For this review, take the finished solid that the model builds, in its own axes (mm). A direction names the side the tool comes from. Coordinates: 2 decimals unless noted, no trailing zeros. Order: outer loops, then holes, each group sorted by start corner. A loop starts at its lowest first (then second) coordinate and runs counter-clockwise, first axis right, second up. Notation, with made-up numbers: M 8.25,-24.75 L 24.25,-24.75 A18 ccw 24.25,-4.75 Z; hole C 19.25,-16 d10. An arc over 180 degrees is marked long. Use one line per item in the form item = value. Start each with the question number.
```python
from build123d import *

# Parameters (mm, degrees)
BOSS_EXTRUDE1_DEPTH = 15
BOSS_EXTRUDE2_DEPTH = 15
SKETCH3_W           = 12
SKETCH3_H           = 4.2
BOSS_EXTRUDE3_DEPTH = 15
CUT_EXTRUDE1_REACH  = 69
SKETCH4_R           = 3.15


with BuildPart() as part:
    # Sketch1 → Boss-Extrude1 (new body)
    with BuildSketch(Plane.XY):
        Polygon((-15, -15), (-15, -4.085), (-13, -2.085), (-17, -2.085), (-17, -17), (17, -17), (17, -2.085), (13, -2.085), (13, -4.085), (15, -4.085), (15, -15), align=None)
    extrude(amount=BOSS_EXTRUDE1_DEPTH)

    # Sketch2 → Boss-Extrude2 (add)
    with BuildSketch(Plane(origin=(0, 0, 0), x_dir=(-1, 0, 0), z_dir=(0, 0, -1))):
        Polygon((-80, 50), (-17, -2.085), (-17, -4.68000212), (-48.089133488, 21.022815621), (-51.622859883, 16.748556949), (-17, -14.313094489), (-17, -17), (-87, 45.8), (-87, 50), (-85, 50), (-85, 45.8), (-84, 45.8), (-84, 50), align=None)
        Polygon((-80.719691535, 48), (-49.630558047, 22.297182259), (-53.112776785, 18.085225255), (-82, 44.001191225), (-82, 48), align=None, mode=Mode.SUBTRACT)
    extrude(amount=-BOSS_EXTRUDE2_DEPTH)

    # Sketch3 → Boss-Extrude3 (add)
    with BuildSketch(Plane(origin=(0, 0, 0), x_dir=(-1, 0, 0), z_dir=(0, 0, -1))):
        with Locations((-93, 47.9)):
            Rectangle(SKETCH3_W, SKETCH3_H)
    extrude(amount=-BOSS_EXTRUDE3_DEPTH)

    # Sketch4 → Cut-Extrude1 (cut, up to next)
    with BuildSketch(Plane(origin=(0, 50, 0), x_dir=(1, 0, 0), z_dir=(0, 1, 0)), mode=Mode.PRIVATE) as cut_extrude1_sk1:
        with Locations((93, -7.5)):
            Circle(SKETCH4_R)
    cut_extrude1_tool1 = extrude(cut_extrude1_sk1.sketch, amount=-CUT_EXTRUDE1_REACH, mode=Mode.PRIVATE) & part.part
    add(cut_extrude1_tool1.solids().sort_by_distance((93, 50, 7.5))[0], mode=Mode.SUBTRACT)


solid = part.part
```
1. For pin 1 Ø3.5 at (y, z) = (-7.5, 4) entering from +X; pin 2 Ø2 at (x, z) = (15.5, 5) entering from +Y (3 decimals); pin 3 Ø8 at (y, z) = (13, 8) entering from -X, all flat-tipped, find the tip position at first contact; note any pin that passes through.
2. To check wall thickness, follow line 1 (Z direction, x = 93, y = 46.7); line 2 (X direction, y = 47.8, z = 7.5); line 3 (X direction, y = 49.1, z = 7.5). State the ranges of each line that lie inside material, in increasing order.
3. The part is to be moulded in two halves that separate along Z. For faces 1 (the flat face through (82, 50, 7)), 2 (the cylindrical face through (89.853, 47.929, 7.362)), 3 (the flat face through (41, 17, 15)), say which applies: pulls with the +Z half, pulls with the -Z half, needs draft (parallel to the pull), parting line crosses it, or undercut.
4. Tool access review of faces 4 (the flat face through (82, 46, 7)), 5 (the flat face through (99, 48, 7)), 6 (the flat face through (-17, -9, 7)), 7 (the flat face through (15, -2.085, 7)): name each direction out of +Z, -Z, +X, -X, +Y, -Y from which nothing blocks a thin tool from reaching the whole face with its end or side.
5. Consider section D-D, the plane y = 15.5. Write out the cut boundary in (x, z), plus the area to 3 significant figures.
6. Consider section B-B, the plane x = 93. Write out the cut boundary in (y, z).
7. Consider section C-C, the plane z = 13.75. Write out the cut boundary in (x, y) (3 decimals).
8. Consider section A-A, the plane z = 7.5. Give the number of separate pieces and of enclosed holes in the cut face, plus the area to 3 significant figures.
Answers follow:
q1.pin_1 = 29.54
q1.pin_2 = -2.085
q1.pin_3 = 30.41
q2.line_1 = 0 to 4.35, 10.65 to 15
q2.line_2 = 77.34 to 80.48, 82 to 84, 85 to 89.85, 96.15 to 99
q2.line_3 = 78.91 to 84, 85 to 89.85, 96.15 to 99
q3.face_1 = needs draft
q3.face_2 = undercut
q3.face_3 = pulls with the +Z half
q4.face_4 = +Z, -Z
q4.face_5 = +Z, -Z, +X, +Y, -Y
q4.face_6 = +Z, -Z, -X, +Y, -Y
q4.face_7 = +Z, -Z, -X, +Y
q5.outline = M 38.27,0 L 41.41,0 L 41.41,15 L 38.27,15 Z; M 50.23,0 L 53.23,0 L 53.23,15 L 50.23,15 Z
q5.area = 92.0 mm²
q6.outline = M 45.8,0 L 50,0 L 50,4.35 L 45.8,4.35 Z; M 45.8,10.65 L 50,10.65 L 50,15 L 45.8,15 Z
q7.outline = M -17,-17 L 17,-17 L 87,45.8 L 99,45.8 L 99,50 L 85,50 L 85,45.8 L 84,45.8 L 84,50 L 80,50 L 17,-2.085 L 13,-2.085 L 13,-4.085 L 15,-4.085 L 15,-15 L -15,-15 L -15,-4.085 L -13,-2.085 L -17,-2.085 Z; hole M 17,-14.313 L 51.623,16.749 L 48.089,21.023 L 17,-4.68 Z; hole M 49.631,22.297 L 53.113,18.085 L 82,44.001 L 82,48 L 80.72,48 Z
q8.separate_pieces = 2
q8.enclosed_holes = 2
q8.area = 531 mm²
